```python
from build123d import *

# Parameters (mm, degrees)
EXTRUDE2_DEPTH = 110.49


with BuildPart() as part:
    # Sketch9 → Extrude2 (new body)
    with BuildSketch(Plane.XY):
        with BuildLine():
            ThreePointArc((-6.35, 0), (95.265102475, 101.615102475), (196.880204949, 0))
            Line((196.880204949, 0), (196.880204949, -6.35))
            Line((196.880204949, -6.35), (190.530204949, -6.35))
            Line((190.530204949, -6.35), (-6.35, -6.35))
            Line((-6.35, -6.35), (-6.35, 0))
        make_face()
        with BuildLine():
            Line((0, 0), (190.530204949, 0))
            ThreePointArc((190.530204949, 0), (95.265102475, 95.265102475), (0, 0))
        make_face(mode=Mode.SUBTRACT)
    extrude(amount=-EXTRUDE2_DEPTH)


solid = part.part
```
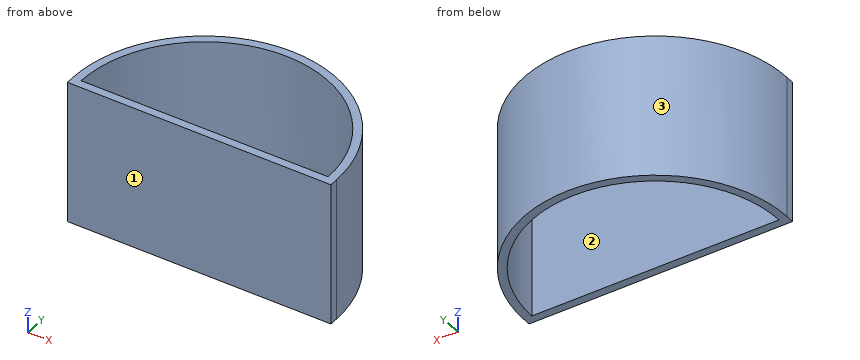
Input: part model. Units: mm. Frame: model coordinates. Face numbers are marked on the shaded views. Give positions to 0.01 mm unless a question says otherwise; leave off trailing zeros. Loops run counter-clockwise (first coordinate to the right, second up) from the corner with the lowest first, then second, coordinate; pieces in that order, holes last. Notation, with made-up numbers: (76, 25.5) -> (102, 25.5) arc R18 ccw to (102, 52.5) -> close; hole circle Ø10 at (8.5, 23). An arc over 180 degrees is marked (long way). Use a Markdown table: item, result.
Q1. Section query C-C, the plane x = 162.5. Return the cut outline in (y, z).
Entries:
| item | result |
|---|---|
| outline | (-6.35, -110.49) -> (0, -110.49) -> (0, 0) -> (-6.35, 0) -> close; (67.49, -110.49) -> (76.19, -110.49) -> (76.19, 0) -> (67.49, 0) -> close |
Q2. Section query A-A, the plane y = 9. Return the cut outline in (x, z), plus the area to 3 significant figures.
Entries:
| item | result |
|---|---|
| outline | (-5.95, -110.49) -> (0.43, -110.49) -> (0.43, 0) -> (-5.95, 0) -> close; (190.1, -110.49) -> (196.48, -110.49) -> (196.48, 0) -> (190.1, 0) -> close |
| area | 1,410 mm² |
Q3. Ray query, probe 1 along Y at (x, z) = (81, -49); probe 2 along X at (y, z) = (55, -98); probe 3 along Y at (x, z) = (105.5, -14.5). Return the intervals inside material, ascending. Write a range as from..to.
Entries:
| item | result |
|---|---|
| probe 1 | y = -6.35..0, 94.19..100.61 |
| probe 2 | x = 9.82..17.48, 173.05..180.71 |
| probe 3 | y = -6.35..0, 94.71..101.1 |
Q4. First-contact query: P1, Ø1, axis at y = 82, z = -79.5, coming from the -X side; P2, Ø8, axis at x = 108.5, z = -58, coming from the +Y side; P3, Ø1, axis at y = 44, z = -78, coming from the +X side. Flat tips, straight axial feed; report the tip coordinate or a pass-through.
Entries:
| item | result |
|---|---|
| P1 | stops at x = 34.57 |
| P2 | stops at y = 101.19 |
| P3 | stops at x = 187.1 |
Q5. Pull-direction query (X, two-part tool) for the marked faces 1, 2 and 3; classes: pulls with the +X half, pulls with the -X half, needs draft (parallel to the pull), parting line crosses it, or undercut.
Entries:
| item | result |
|---|---|
| face 1 | needs draft |
| face 2 | undercut |
| face 3 | parting line crosses it |
Q6. Section query B-B, the plane z = -56.5. Return the cut outline in (x, y).
Entries:
| item | result |
|---|---|
| outline | (-6.35, -6.35) -> (196.88, -6.35) -> (196.88, 0) arc R101.62 ccw to (-6.35, 0) -> close; hole (0, 0) -> (190.53, 0) arc R95.27 ccw to start |
